Geometry: final body of the model. Coordinates: model frame, mm. A direction names the side the tool comes from. Round coordinates to 2 decimals unless told otherwise and drop trailing zeros. Loops run counter-clockwise (first coordinate to the right, second up) from the corner with the lowest first, then second, coordinate; pieces in that order, holes last. Notation, with made-up numbers: (57.5, 40.5) - (88.5, 40.5) arc R24 cw to (88.5, 63.5) - close; hole circle Ø9 at (-3, 70). An arc over 180 degrees is marked (long way). Use CSV: the item, a comma, the result in double quotes.
from build123d import *

# Parameters (mm, degrees)
F0_R     = 29.845
F0_R_2   = 25.4
F1_DEPTH = 50.8
F2_R     = 44.45
F3_DEPTH = 12.7
F4_R     = 5.08
F6_D     = 50.8
F7_R     = 44.45
F8_DEPTH = 12.7
F9_R     = 5.08
F11_D    = 50.8


with BuildPart() as f1:
    # F0 (on Top) → F1 (new body, symmetric)
    with BuildSketch(Plane.XY):
        Circle(F0_R)
        Circle(F0_R_2, mode=Mode.SUBTRACT)
    extrude(amount=F1_DEPTH, both=True)

    # F2 (on face) → F3 (join)
    with BuildSketch(Plane(origin=(0, 0, -50.8), x_dir=(1, 0, 0), z_dir=(0, 0, -1))):
        Circle(F2_R)
    extrude(amount=-F3_DEPTH)

    # F4
    f4_edges = [f1.edges().sort_by_distance(p)[0] for p in [
        (44.45, 0, -44.45),
        (-44.45, 0, -50.8),
        (-44.45, 0, -38.1),
    ]]
    fillet(f4_edges, radius=F4_R)

    # F6 (through all)
    with Locations(Plane(origin=(0, 0, -50.8), x_dir=(1, 0, 0), z_dir=(0, 0, -1))):
        with Locations((0, 0)):
            Hole(F6_D / 2)

    # F7 (on face) → F8 (join)
    with BuildSketch(Plane.XY.offset(50.8)):
        Circle(F7_R)
    extrude(amount=-F8_DEPTH)

    # F9
    f9_edges = [f1.edges().sort_by_distance(p)[0] for p in [
        (44.45, 0, 44.45),
        (-44.45, 0, 50.8),
        (-44.45, 0, 38.1),
    ]]
    fillet(f9_edges, radius=F9_R)

    # F11 (through all)
    with Locations(Plane.XY.offset(50.8)):
        with Locations((0, 0)):
            Hole(F11_D / 2)


solid = f1.part
Item 1: Mould query, pull axis Z, two halves, no side actions, for faces 1 (the cylindrical face through (42.397, 13.352, 44.468)), 2 (the cylindrical face through (28.47, 8.96, 0.53)), 3 (the flat face through (-1, 26, -50.8)). Classes: released by +Z, released by -Z, zero draft, split by the parting line, or undercut.
Final values:
face 1,"zero draft"
face 2,"undercut"
face 3,"released by -Z"
Item 2: Section B-B on z = 34.5. Return the cut outline in (x, y) (3 decimals).
Final values:
outline,"circle Ø59.69 at (0, 0); hole circle Ø50.8 at (0, 0)"
Item 3: Section A-A on x = 0. Return the cut outline in (y, z) (3 decimals), plus the area to 3 significant figures.
Final values:
outline,"(-44.45, -45.72) arc R5.08 ccw to (-39.37, -50.8) - (-25.4, -50.8) - (-25.4, 50.8) - (-39.37, 50.8) arc R5.08 ccw to (-44.45, 45.72) - (-44.45, 43.18) arc R5.08 ccw to (-39.37, 38.1) - (-29.845, 38.1) - (-29.845, -38.1) - (-39.37, -38.1) arc R5.08 ccw to (-44.45, -43.18) - close; (25.4, -50.8) - (39.37, -50.8) arc R5.08 ccw to (44.45, -45.72) - (44.45, -43.18) arc R5.08 ccw to (39.37, -38.1) - (29.845, -38.1) - (29.845, 38.1) - (39.37, 38.1) arc R5.08 ccw to (44.45, 43.18) - (44.45, 45.72) arc R5.08 ccw to (39.37, 50.8) - (25.4, 50.8) - close"
area,"1,600 mm²"
Item 4: Reachability of faces 4 (the flat face through (14.4, 26.4, 38.1)), 5 (the cylindrical face through (42.397, -13.352, -44.468)) from +Z, -Z, +X, -X, +Y, -Y: full face, straight path, thin tool, end or side. Return the list, or none.
Final values:
face 4,"none"
face 5,"+Z, -Z"
Item 5: Pin query (flat end, axial travel): P1, Ø4, axis at x = -2, z = 16.5, coming from the -Y side (3 decimals); P2, Ø10, axis at y = 29, z = -14.5, coming from the -X side; P3, Ø10, axis at x = 29.5, z = 26, coming from the -Y side. Return the tip coordinate at first contact, or that it passes through.
Final values:
P1,"stops at y = -29.845"
P2,"stops at x = -17.74"
P3,"stops at y = -17.04"
Item 6: Material intervals for line 1 (Y direction, x = 0, z = 43); line 2 (Z direction, x = 4, y = 36); line 3 (X direction, y = -1, z = 37.5), sorted ascending.
Final values:
line 1,"y = -44.45 to -25.4, 25.4 to 44.45"
line 2,"z = -50.8 to -38.1, 38.1 to 50.8"
line 3,"x = -29.83 to -25.38, 25.38 to 29.83"
